```python
from build123d import *

# Parameters (mm, degrees)
EXTRUSION1_DEPTH = 11
ESQUISSE2_R      = 3.11
EXTRUSION2_DEPTH = 27.424530578
ESQUISSE3_R      = 1.5
EXTRUSION3_DEPTH = 11


with BuildPart() as part:
    # Esquisse1 → Extrusion1 (new body)
    with BuildSketch(Plane.XY):
        Polygon((-11.094787824, -6.686254611), (-11.094787824, 13.313745389), (-9.594787824, 13.313745389), (-9.594787824, -5.186254611), (7.405212176, -5.186254611), (7.405212176, 13.313745389), (8.905212176, 13.313745389), (8.905212176, -6.686254611), align=None)
    extrude(amount=EXTRUSION1_DEPTH)

    # Esquisse2 → Extrusion2 (cut, through all)
    with BuildSketch(Plane(origin=(8.905212176, 0, 0), x_dir=(0, 0, -1), z_dir=(1, 0, 0))):
        with Locations((-5.5, 2.313745389)):
            Circle(ESQUISSE2_R)
    extrude(amount=-EXTRUSION2_DEPTH, mode=Mode.SUBTRACT)

    # Esquisse3 → Extrusion3 (cut)
    with BuildSketch(Plane(origin=(0, -5.186254611, 0), x_dir=(-1, 0, 0), z_dir=(0, 1, 0))):
        with Locations(Location((5.094787824, 5.5, 0), (0, 0, 90))):
            Circle(ESQUISSE3_R)
        with Locations(Location((-2.905212176, 5.5, 0), (0, 0, 90))):
            Circle(ESQUISSE3_R)
    extrude(amount=-EXTRUSION3_DEPTH, mode=Mode.SUBTRACT)


solid = part.part
```
Geometry: final body of the model. Coordinates: model frame, mm. A direction names the side the tool comes from. Round coordinates to 2 decimals unless told otherwise and drop trailing zeros. Loops run counter-clockwise (first coordinate to the right, second up) from the corner with the lowest first, then second, coordinate; pieces in that order, holes last. Notation, with made-up numbers: (80.5, -18) -> (108.5, -18) arc R22 ccw to (108.5, -12) -> close; hole circle Ø8 at (38.5, 85.25). An arc over 180 degrees is marked (long way). Use one line per item in the form item = value.
Item 1: Contact query for flat-ended pins moving along their axis: pin 1 Ø1.5 at (x, z) = (0, 3) entering from +Y; pin 2 Ø2.5 at (x, z) = (-5.09, 5.5) entering from -Y; pin 3 Ø12 at (x, y) = (4, -1) entering from -Z. Output: stop coordinate, or through.
Evaluation:
pin_1 = -5.19
pin_2 = through
pin_3 = 0
Item 2: Access query for faces 1 (the cylindrical face through (-6.01, -5.93, 4.31)), 2 (the flat face through (-1, -5.186, 5)). Directions: +Z, -Z, +X, -X, +Y, -Y. A direction counts if a zero-diameter tool reaches every point of the face in a straight line with its end or side. Return the directions, or none.
Evaluation:
face_1 = +Y, -Y
face_2 = +Z, -Z, +Y
Item 3: Material intervals for probe 1 along X at (y, z) = (-5.5, 5.5); probe 2 along X at (y, z) = (-4, 4.5); probe 3 along Y at (x, z) = (7.85, 5.5), sorted ascending.
Evaluation:
probe_1 = -11.09 to -6.59, -3.59 to 1.41, 4.41 to 8.91
probe_2 = -11.09 to -9.59, 7.41 to 8.91
probe_3 = -6.69 to -0.8, 5.42 to 13.31
Item 4: Cut plane B-B on y = -4.25. Output: boundary loops of the cut face in (x, z), then the cut area to 3 significant figures.
Evaluation:
outline = (-11.09, 0) -> (-9.59, 0) -> (-9.59, 11) -> (-11.09, 11) -> close; (7.41, 0) -> (8.91, 0) -> (8.91, 11) -> (7.41, 11) -> close
area = 33.0 mm2
Item 5: Cut plane C-C on z = 7.25. Output: boundary loops of the cut face in (x, y), then the cut area to 3 significant figures.
Evaluation:
outline = (-11.09, -6.69) -> (8.91, -6.69) -> (8.91, -0.26) -> (7.41, -0.26) -> (7.41, -5.19) -> (-9.59, -5.19) -> (-9.59, -0.26) -> (-11.09, -0.26) -> close; (-11.09, 4.88) -> (-9.59, 4.88) -> (-9.59, 13.31) -> (-11.09, 13.31) -> close; (7.41, 4.88) -> (8.91, 4.88) -> (8.91, 13.31) -> (7.41, 13.31) -> close
area = 70.1 mm2
Item 6: Cut plane A-A on z = 5.5. Output: boundary loops of the cut face in (x, y).
Evaluation:
outline = (-11.09, -6.69) -> (-6.59, -6.69) -> (-6.59, -5.19) -> (-9.59, -5.19) -> (-9.59, -0.8) -> (-11.09, -0.8) -> close; (-11.09, 5.42) -> (-9.59, 5.42) -> (-9.59, 13.31) -> (-11.09, 13.31) -> close; (-3.59, -6.69) -> (1.41, -6.69) -> (1.41, -5.19) -> (-3.59, -5.19) -> close; (4.41, -6.69) -> (8.91, -6.69) -> (8.91, -0.8) -> (7.41, -0.8) -> (7.41, -5.19) -> (4.41, -5.19) -> close; (7.41, 5.42) -> (8.91, 5.42) -> (8.91, 13.31) -> (7.41, 13.31) -> close
Item 7: Cut plane D-D on x = -5.75. Output: boundary loops of the cut face in (y, z).
Evaluation:
outline = (-6.69, 0) -> (-5.19, 0) -> (-5.19, 4.15) -> (-6.69, 4.15) -> close; (-6.69, 6.85) -> (-5.19, 6.85) -> (-5.19, 11) -> (-6.69, 11) -> close
Item 8: Draft query along Y for faces 3 (the cylindrical face through (8.166, 3.248, 2.534)), 4 (the flat face through (-1, -6, 0)), 5 (the flat face through (8, 13.314, 5)), 6 (the cylindrical face through (-10.334, 3.248, 2.534)). Return one class per face: released by +Y, released by -Y, zero draft, split by the parting line, or undercut.
Evaluation:
face_3 = undercut
face_4 = zero draft
face_5 = released by +Y
face_6 = undercut
